Answer from the drawing. Dimensions are ordinates in mm from the lowest x, y and z of the part. Round coordinates to 2 decimals unless told otherwise and drop trailing zeros. Loops run counter-clockwise (first coordinate to the right, second up) from the corner with the lowest first, then second, coordinate; pieces in that order, holes last. Notation, with made-up numbers: M 48,43 L 101,43 A8 ccw 101,54 Z; hole C -3.75,67.25 d9. An arc over 180 degrees is marked long. Answer as a JSON object with one key per item and string values.
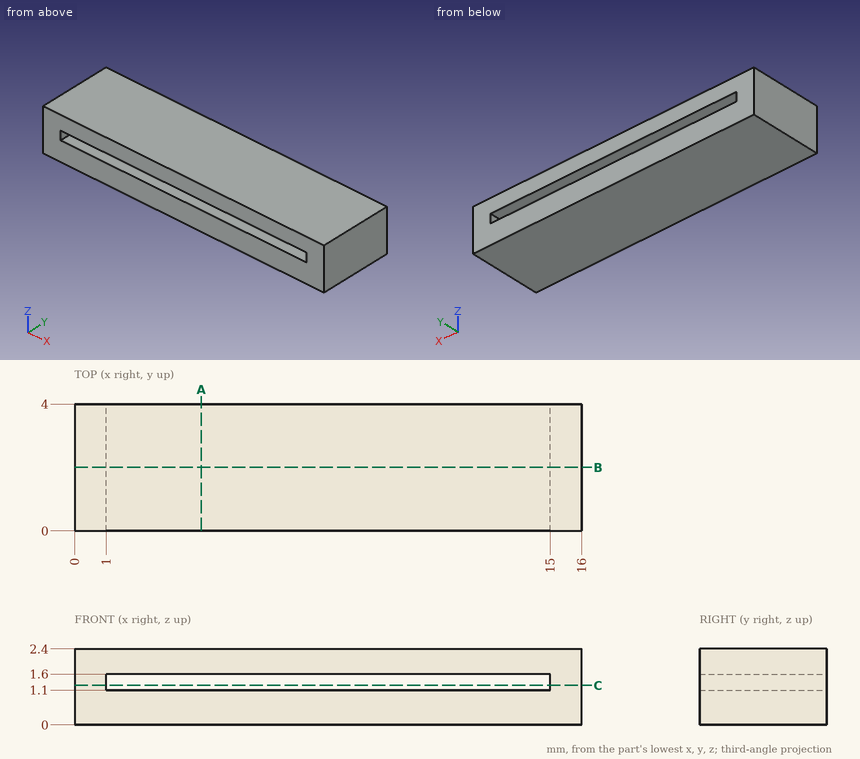
Item 1: The part is cut by section C-C (z = 1.25). Give the vertices of the cut face in (x, y), then the cut area to 3 significant figures.
Values follow:
{"outline": "M 0,0 L 1,0 L 1,4 L 0,4 Z; M 15,0 L 16,0 L 16,4 L 15,4 Z", "area": "8.00 mm^2"}
Item 2: Straight lines are drawn through the part: line 1 (Z direction, x = 4.5, y = 0.95); line 2 (X direction, y = 1.3, z = 1.5). For each, find the intervals that lie inside material, in ascending order.
Values follow:
{"line 1": "0 to 1.1, 1.6 to 2.4", "line 2": "0 to 1, 15 to 16"}
Item 3: The part is cut by section B-B (y = 2). Give the vertices of the cut face in (x, z), then the cut area to 3 significant figures.
Values follow:
{"outline": "M 0,0 L 16,0 L 16,2.4 L 0,2.4 Z; hole M 1,1.1 L 15,1.1 L 15,1.6 L 1,1.6 Z", "area": "31.4 mm^2"}
Item 4: The part is cut by section A-A (x = 4). Give the vertices of the cut face in (y, z).
Values follow:
{"outline": "M 0,0 L 4,0 L 4,1.1 L 0,1.1 Z; M 0,1.6 L 4,1.6 L 4,2.4 L 0,2.4 Z"}
